Could you check a few things on this model? Use its own coordinates, in mm. Face numbers are marked on the shaded views. Coordinates: 2 decimals unless noted, no trailing zeros. Loops run counter-clockwise (first coordinate to the right, second up) from the corner with the lowest first, then second, coordinate; pieces in that order, holes last.
1) Imagine slicing it at C-C on z = 5. Please give me the cut outline in (x, y), plus the area to 3 significant figures.
2) Thinking about a two-plate mould opening in X: for the marked faces 1 and 2, which applies, released by +X, released by -X, zero draft, split by the parting line, or undercut?
3) Imagine slicing it at B-B on x = 52. Please give me the cut outline in (y, z).
4) Imagine slicing it at D-D on x = 14. Please give me the cut outline in (y, z).
5) Will these pins go through, and if not, where does the flat tip stop? P1, Ø1.8, axis at y = 6.5, z = -7.5, coming from the +X side; P2, Ø8, axis at x = 3, z = 6, coming from the +Y side; P3, Ø1.8, axis at y = 5, z = -8, coming from the -X side.
6) If I drill on line 1 along X through (y, z) = (4.25, -1); line 2 along Y through (x, z) = (-31, -42); line 3 along Z through (x, y) = (66, 3.75), over which ranges is the centre line in solid material (lowest first)?
7) Imagine slicing it at A-A on y = 4.5. Please give me the cut outline in (x, z), plus the area to 3 significant figures.
```python
from build123d import *

# Parameters (mm, degrees)
SKETCH1_W           = 149.86
SKETCH1_H           = 116.84
BOSS_EXTRUDE1_DEPTH = 2
FILLET1_R           = 7.62
SKETCH2_W           = 19.05
SKETCH2_H           = 78.74
BOSS_EXTRUDE2_DEPTH = 5.842


with BuildPart() as part:
    # Sketch1 → Boss-Extrude1 (new body)
    with BuildSketch(Plane(origin=(0, 0, 0), x_dir=(1, 0, 0), z_dir=(0, 1, 0))):
        Rectangle(SKETCH1_W, SKETCH1_H)
    extrude(amount=BOSS_EXTRUDE1_DEPTH)

    # Fillet1
    fillet1_edges = [part.edges().sort_by_distance(p)[0] for p in [
        (-74.93, 1, -58.42),
        (74.93, 1, -58.42),
        (74.93, 1, 58.42),
        (-74.93, 1, 58.42),
    ]]
    fillet(fillet1_edges, radius=FILLET1_R)

    # Sketch2 → Boss-Extrude2 (add)
    with BuildSketch(Plane(origin=(0, 2, 0), x_dir=(1, 0, 0), z_dir=(0, 1, 0))):
        with Locations((59.055, -7.62)):
            Rectangle(SKETCH2_W, SKETCH2_H)
    boss_extrude2 = extrude(amount=BOSS_EXTRUDE2_DEPTH)

    # Mirror1: Boss-Extrude2 across plane
    add(boss_extrude2.mirror(Plane(origin=(0, 0, 0), x_dir=(0, 0, 1), z_dir=(1, 0, 0))))


solid = part.part
```
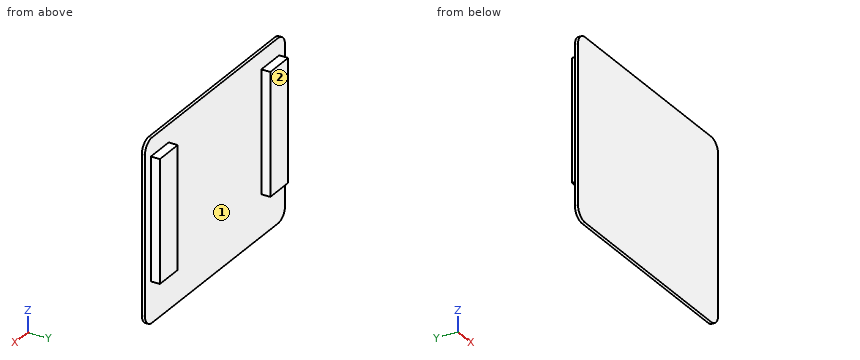
Filled in:
1. outline: (-74.93, 0) - (74.93, 0) - (74.93, 2) - (68.58, 2) - (68.58, 7.84) - (49.53, 7.84) - (49.53, 2) - (-49.53, 2) - (-49.53, 7.84) - (-68.58, 7.84) - (-68.58, 2) - (-74.93, 2) - close
1. area: 522 mm2
2. face 1: undercut
2. face 2: zero draft
3. outline: (0, -58.42) - (2, -58.42) - (2, -31.75) - (7.84, -31.75) - (7.84, 46.99) - (2, 46.99) - (2, 58.42) - (0, 58.42) - close
4. outline: (0, -58.42) - (2, -58.42) - (2, 58.42) - (0, 58.42) - close
5. P1: stops at x = 68.58
5. P2: stops at y = 2
5. P3: stops at x = -68.58
6. line 1: x = -68.58 to -49.53, 49.53 to 68.58
6. line 2: y = 0 to 2
6. line 3: z = -31.75 to 46.99
7. outline: (-68.58, -31.75) - (-49.53, -31.75) - (-49.53, 46.99) - (-68.58, 46.99) - close; (49.53, -31.75) - (68.58, -31.75) - (68.58, 46.99) - (49.53, 46.99) - close
7. area: 3,000 mm2
